from build123d import *


with BuildPart() as part:
    # Эскиз1 → Повернуть1 (revolve)
    with BuildSketch(Plane(origin=(0, 0, 0), x_dir=(0, 0, -1), z_dir=(1, 0, 0))):
        Polygon((20, 30), (20, 26), (5, 26), (5, 21), (0, 21), (0, 30), align=None)
    revolve(axis=Axis((0, 0, 1000), (0, 0, -1)))

    # Зеркальное отражение1: part across plane


with BuildPart() as part_1:
    add(part.part)
    add(part.part.mirror(Plane(origin=(0, 21, 0), x_dir=(1, 0, 0), z_dir=(0, 0, -1))))


solid = part_1.part
Source: CAD feature listing. Evaluate the final solid. Frame: model axes, mm. A direction names the side the tool comes from. Round coordinates to 2 decimals unless told otherwise and drop trailing zeros. Write each loop counter-clockwise with the first axis right and the second up, starting at its lowest first coordinate (ties: lowest second). Pieces come first, ordered by that corner, then holes. Notation, with made-up numbers: (66.5, 37.5) - (97.5, 37.5) arc R16 ccw to (97.5, 65.5) - close; hole circle Ø10 at (3.25, 76.25). An arc over 180 degrees is marked (long way). Use CSV: the item, a comma, the result in double quotes. Start each with the question number.
(1) Material intervals for probe 1 along X at (y, z) = (0, -1.5); probe 2 along X at (y, z) = (0, 11.5); probe 3 along Z at (x, y) = (5, -25), sorted ascending. Write a range as [from, to].
(2) Cut plane D-D, the plane y = 23. Return loops of the section in (x, z), and give its area (3 significant figures).
(3) Set-up query: faces 5 (the face through (25, -9, 20)), 6 (the face through (-15.821, -20.633, 12.395)). Return all of +Z, -Z, +X, -X, +Y, -Y with unobstructed straight access to the full face (end or side cutting, diameter ignored); none if empty.
(4) Mould query, pull axis Y, two halves, no side actions, for faces 1 (the face through (1.32, -29.97, 0.28)), 2 (the face through (-15.821, -20.633, -12.395)), 3 (the face through (21.3, 1.8, -5)), 4 (the face through (25, -9, -20)). Classes: pulls with the +Y half, pulls with the -Y half, needs draft (parallel to the pull), parting line crosses it, or undercut.
(5) First-contact query: pin 1 Ø1.5 at (y, z) = (-14, 9.5) entering from -X; pin 2 Ø2 at (y, z) = (-6.5, 7.5) entering from -X; pin 3 Ø10 at (y, z) = (-6.5, 1) entering from +X. Flat tips, straight axial feed; report the tip coordinate or a pass-through.
(6) Cut plane A-A, the plane y = 0. Return loops of the section in (x, z), and give its area (3 significant figures).
(7) Cut plane C-C, the plane z = 11. Return loops of the section in (x, y), and give its area (3 significant figures).
Geometry says:
1,probe 1,"[-30, -21], [21, 30]"
1,probe 2,"[-30, -26], [26, 30]"
1,probe 3,"[-5, 5]"
2,outline,"(-19.26, -20) - (-12.12, -20) - (-12.12, -5) - (12.12, -5) - (12.12, -20) - (19.26, -20) - (19.26, 20) - (12.12, 20) - (12.12, 5) - (-12.12, 5) - (-12.12, 20) - (-19.26, 20) - close"
2,area,"813 mm²"
3,face 5,"+Z, +X, -X, +Y, -Y"
3,face 6,"+Z"
4,face 1,"parting line crosses it"
4,face 2,"undercut"
4,face 3,"undercut"
4,face 4,"needs draft"
5,pin 1,"x = -26.92"
5,pin 2,"x = -29.49"
5,pin 3,"x = 29.96"
6,outline,"(-30, -20) - (-26, -20) - (-26, -5) - (-21, -5) - (-21, 5) - (-26, 5) - (-26, 20) - (-30, 20) - close; (21, -5) - (26, -5) - (26, -20) - (30, -20) - (30, 20) - (26, 20) - (26, 5) - (21, 5) - close"
6,area,"420 mm²"
7,outline,"circle Ø60 at (0, 0); hole circle Ø52 at (0, 0)"
7,area,"704 mm²"
